The model under review builds one solid part; all positions refer to its coordinate system, in mm. Round coordinates to 2 decimals unless told otherwise and drop trailing zeros. Order: outer loops, then holes, each group sorted by start corner. A loop starts at its lowest first (then second) coordinate and runs counter-clockwise, first axis right, second up. Notation, with made-up numbers: (46, -17.5) -> (103, -17.5) arc R6 ccw to (103, -10.5) -> close; hole circle Ø4 at (86, 57). An arc over 180 degrees is marked (long way). Use a Markdown table: item, result. Add a question column.
```python
from build123d import *

# Parameters (mm, degrees)
SKETCH1_R           = 250
SKETCH1_R_2         = 5.1
SKETCH1_R_3         = 12.5
SKETCH1_R_4         = 1.6
BOSS_EXTRUDE1_DEPTH = 2.5


with BuildPart() as part:
    # Sketch1 → Boss-Extrude1 (new, symmetric)
    with BuildSketch(Plane(origin=(0, 0, 0), x_dir=(1, 0, 0), z_dir=(0, 1, 0))):
        with Locations(Location((0, 0, 0), (0, 0, 270))):
            Circle(SKETCH1_R)
        with Locations(Location((0, 222.5, 0), (0, 0, 270))):
            Circle(SKETCH1_R_2, mode=Mode.SUBTRACT)
        with Locations(Location((192.690652342, 111.25, 0), (0, 0, 270))):
            Circle(SKETCH1_R_2, mode=Mode.SUBTRACT)
        with Locations(Location((192.690652342, -111.25, 0), (0, 0, 270))):
            Circle(SKETCH1_R_2, mode=Mode.SUBTRACT)
        with Locations(Location((0, -222.5, 0), (0, 0, 270))):
            Circle(SKETCH1_R_2, mode=Mode.SUBTRACT)
        with Locations(Location((-192.690652342, -111.25, 0), (0, 0, 270))):
            Circle(SKETCH1_R_2, mode=Mode.SUBTRACT)
        with Locations(Location((-192.690652342, 111.25, 0), (0, 0, 270))):
            Circle(SKETCH1_R_2, mode=Mode.SUBTRACT)
        with Locations(Location((0, 0, 0), (0, 0, 270))):
            Circle(SKETCH1_R_3, mode=Mode.SUBTRACT)
        with Locations(Location((-10, 100.754962657, 0), (0, 0, 270))):
            Circle(SKETCH1_R_4, mode=Mode.SUBTRACT)
        with Locations(Location((10, 100.754962657, 0), (0, 0, 270))):
            Circle(SKETCH1_R_4, mode=Mode.SUBTRACT)
        with Locations(Location((-10.575, 112.738110965, 0), (0, 0, 270))):
            Circle(SKETCH1_R_4, mode=Mode.SUBTRACT)
        with Locations(Location((10.575, 112.738110965, 0), (0, 0, 90))):
            Circle(SKETCH1_R_4, mode=Mode.SUBTRACT)
        with Locations(Location((72.240228551, 87.195536973, 0), (0, 0, 270))):
            Circle(SKETCH1_R_4, mode=Mode.SUBTRACT)
        with Locations(Location((87.195536973, 72.240228551, 0), (0, 0, 90))):
            Circle(SKETCH1_R_4, mode=Mode.SUBTRACT)
        with Locations(Location((78.315585145, 64.173449521, 0), (0, 0, 270))):
            Circle(SKETCH1_R_4, mode=Mode.SUBTRACT)
        with Locations(Location((64.173449521, 78.315585145, 0), (0, 0, 270))):
            Circle(SKETCH1_R_4, mode=Mode.SUBTRACT)
        with Locations(Location((112.738110965, 10.575, 0), (0, 0, 270))):
            Circle(SKETCH1_R_4, mode=Mode.SUBTRACT)
        with Locations(Location((112.738110965, -10.575, 0), (0, 0, 90))):
            Circle(SKETCH1_R_4, mode=Mode.SUBTRACT)
        with Locations(Location((100.754962657, -10, 0), (0, 0, 270))):
            Circle(SKETCH1_R_4, mode=Mode.SUBTRACT)
        with Locations(Location((100.754962657, 10, 0), (0, 0, 270))):
            Circle(SKETCH1_R_4, mode=Mode.SUBTRACT)
        with Locations(Location((87.195536973, -72.240228551, 0), (0, 0, 270))):
            Circle(SKETCH1_R_4, mode=Mode.SUBTRACT)
        with Locations(Location((72.240228551, -87.195536973, 0), (0, 0, 90))):
            Circle(SKETCH1_R_4, mode=Mode.SUBTRACT)
        with Locations(Location((64.173449521, -78.315585145, 0), (0, 0, 270))):
            Circle(SKETCH1_R_4, mode=Mode.SUBTRACT)
        with Locations(Location((78.315585145, -64.173449521, 0), (0, 0, 270))):
            Circle(SKETCH1_R_4, mode=Mode.SUBTRACT)
        with Locations(Location((10.575, -112.738110965, 0), (0, 0, 270))):
            Circle(SKETCH1_R_4, mode=Mode.SUBTRACT)
        with Locations(Location((-10.575, -112.738110965, 0), (0, 0, 90))):
            Circle(SKETCH1_R_4, mode=Mode.SUBTRACT)
        with Locations(Location((-10, -100.754962657, 0), (0, 0, 270))):
            Circle(SKETCH1_R_4, mode=Mode.SUBTRACT)
        with Locations(Location((10, -100.754962657, 0), (0, 0, 270))):
            Circle(SKETCH1_R_4, mode=Mode.SUBTRACT)
        with Locations(Location((-72.240228551, -87.195536973, 0), (0, 0, 270))):
            Circle(SKETCH1_R_4, mode=Mode.SUBTRACT)
        with Locations(Location((-87.195536973, -72.240228551, 0), (0, 0, 90))):
            Circle(SKETCH1_R_4, mode=Mode.SUBTRACT)
        with Locations(Location((-78.315585145, -64.173449521, 0), (0, 0, 270))):
            Circle(SKETCH1_R_4, mode=Mode.SUBTRACT)
        with Locations(Location((-64.173449521, -78.315585145, 0), (0, 0, 270))):
            Circle(SKETCH1_R_4, mode=Mode.SUBTRACT)
        with Locations(Location((-112.738110965, -10.575, 0), (0, 0, 270))):
            Circle(SKETCH1_R_4, mode=Mode.SUBTRACT)
        with Locations(Location((-112.738110965, 10.575, 0), (0, 0, 90))):
            Circle(SKETCH1_R_4, mode=Mode.SUBTRACT)
        with Locations(Location((-100.754962657, 10, 0), (0, 0, 270))):
            Circle(SKETCH1_R_4, mode=Mode.SUBTRACT)
        with Locations(Location((-100.754962657, -10, 0), (0, 0, 270))):
            Circle(SKETCH1_R_4, mode=Mode.SUBTRACT)
        with Locations(Location((-87.195536973, 72.240228551, 0), (0, 0, 270))):
            Circle(SKETCH1_R_4, mode=Mode.SUBTRACT)
        with Locations(Location((-72.240228551, 87.195536973, 0), (0, 0, 90))):
            Circle(SKETCH1_R_4, mode=Mode.SUBTRACT)
        with Locations(Location((-64.173449521, 78.315585145, 0), (0, 0, 270))):
            Circle(SKETCH1_R_4, mode=Mode.SUBTRACT)
        with Locations(Location((-78.315585145, 64.173449521, 0), (0, 0, 270))):
            Circle(SKETCH1_R_4, mode=Mode.SUBTRACT)
    extrude(amount=BOSS_EXTRUDE1_DEPTH, both=True)


solid = part.part
```
Q1. Add section C-C, the plane y = 0.8. Give the number of separate pieces and of enclosed holes in the cut face, then the cut area to 3 significant figures.
Q2. Add section B-B, the plane z = 176. Give the boundary of the cut face in (x, y), then the cut area to 3 significant figures.
Q3. Draft analysis for pull direction X (two halves, no side actions). For faces 1 (the face through (4, -2.5, 52)), 2 (the face through (3.755, -0.035, 11.923)), 3 (the face through (10.99, 0.04, -249.76)), state which applies: released by +X, released by -X, zero draft, split by the parting line, or undercut.
Q4. Add section D-D, the plane x = -204. Give the boundary of the cut face in (y, z).
Q5. To check wall thickness, follow line 1 along Z through (x, y) = (11, -0.9); line 2 along X through (y, z) = (1.7, -2.5); line 3 along Z through (x, y) = (3, -2.1). State the ranges of each line that lie inside material, in increasing order.
Q6. For pin 1 (3 mm diameter, centred on x = 72.24, z = -87.2, fed in from +Y); pin 2 (1.5 mm diameter, centred on x = -121, y = -1, fed in from +Z); pin 3 (1 mm diameter, centred on y = 2, z = -42, fed in from -X); pin 4 (11.5 mm diameter, centred on x = 0, z = 222.5, fed in from +Y), all flat-tipped, find the tip position at first contact; note any pin that passes through.
Q7. Add section A-A, the plane z = 0. Give the boundary of the cut face in (x, y).
Return value:
| question | item | result |
|---|---|---|
| 1 | separate pieces | 1 |
| 1 | enclosed holes | 39 |
| 1 | area | 195,000 mm² |
| 2 | outline | (-177.55, -2.5) -> (177.55, -2.5) -> (177.55, 2.5) -> (-177.55, 2.5) -> close |
| 2 | area | 1,780 mm² |
| 3 | face 1 | zero draft |
| 3 | face 2 | undercut |
| 3 | face 3 | split by the parting line |
| 4 | outline | (-2.5, -144.51) -> (2.5, -144.51) -> (2.5, 144.51) -> (-2.5, 144.51) -> close |
| 5 | line 1 | -249.76 to -114.28, -111.2 to -102, -99.51 to -5.94, 5.94 to 99.51, 102 to 111.2, 114.28 to 249.76 |
| 5 | line 2 | -249.99 to -12.25, 12.25 to 249.99 |
| 5 | line 3 | -249.98 to -226.62, -218.38 to -12.13, 12.13 to 218.38, 226.62 to 249.98 |
| 6 | pin 1 | through |
| 6 | pin 2 | z = 219.18 |
| 6 | pin 3 | x = -246.53 |
| 6 | pin 4 | y = 2.5 |
| 7 | outline | (-250, -2.5) -> (-12.5, -2.5) -> (-12.5, 2.5) -> (-250, 2.5) -> close; (12.5, -2.5) -> (250, -2.5) -> (250, 2.5) -> (12.5, 2.5) -> close |
